from build123d import *

# Parameters (mm, degrees)
SKIZZE1_W                       = 730
SKIZZE1_H                       = 1060
AUFSATZ_LINEAR_AUSTRAGEN1_DEPTH = 21
SKIZZE2_W                       = 17
SKIZZE2_H                       = 1060
SCHNITT_LINEAR_AUSTRAGEN1_DEPTH = 11
SKIZZE3_R                       = 3.5
SCHNITT_LINEAR_AUSTRAGEN2_DEPTH = 40


with BuildPart() as part:
    # Skizze1 → Aufsatz-Linear austragen1 (new body)
    with BuildSketch(Plane.XY):
        Rectangle(SKIZZE1_W, SKIZZE1_H)
    extrude(amount=AUFSATZ_LINEAR_AUSTRAGEN1_DEPTH)

    # Skizze2 → Schnitt-Linear austragen1 (cut)
    with BuildSketch(Plane.XY.offset(21)):
        with Locations((58.5, 0)):
            Rectangle(SKIZZE2_W, SKIZZE2_H)
        with Locations((175.5, 0)):
            Rectangle(SKIZZE2_W, SKIZZE2_H)
        with Locations((292.5, 0)):
            Rectangle(SKIZZE2_W, SKIZZE2_H)
        with Locations((-292.5, 0)):
            Rectangle(SKIZZE2_W, SKIZZE2_H)
        with Locations((-175.5, 0)):
            Rectangle(SKIZZE2_W, SKIZZE2_H)
        with Locations((-58.5, 0)):
            Rectangle(SKIZZE2_W, SKIZZE2_H)
    extrude(amount=-SCHNITT_LINEAR_AUSTRAGEN1_DEPTH, mode=Mode.SUBTRACT)

    # Skizze3 → Schnitt-Linear austragen2 (cut)
    with BuildSketch(Plane.XY.offset(21)):
        with Locations((0, 490)):
            Circle(SKIZZE3_R)
        with Locations((117, 490)):
            Circle(SKIZZE3_R)
        with Locations((234, 490)):
            Circle(SKIZZE3_R)
        with Locations((340, 490)):
            Circle(SKIZZE3_R)
        with Locations((340, 190)):
            Circle(SKIZZE3_R)
        with Locations((234, 190)):
            Circle(SKIZZE3_R)
        with Locations((117, 190)):
            Circle(SKIZZE3_R)
        with Locations((0, 190)):
            Circle(SKIZZE3_R)
        with Locations(Location((-340, 490, 0), (0, 0, 180))):
            Circle(SKIZZE3_R)
        with Locations(Location((-234, 490, 0), (0, 0, 180))):
            Circle(SKIZZE3_R)
        with Locations(Location((-117, 490, 0), (0, 0, 180))):
            Circle(SKIZZE3_R)
    extrude(amount=-SCHNITT_LINEAR_AUSTRAGEN2_DEPTH, mode=Mode.SUBTRACT)


solid = part.part
Can you work these out from the model? Positions are in its coordinate system, mm. Round coordinates to 2 decimals unless told otherwise and drop trailing zeros. Write each loop counter-clockwise with the first axis right and the second up, starting at its lowest first coordinate (ties: lowest second). Pieces come first, ordered by that corner, then holes. Notation, with made-up numbers: M 18,29.25 L 27,29.25 A18 ccw 27,51.25 Z; hole C 27,-14 d2. An arc over 180 degrees is marked long. Use CSV: the item, a comma, the result in double quotes.
(1) I need wall thicknesses on line 1 along Y through (x, z) = (117, 15.5); line 2 along Y through (x, z) = (-234, 6.75); line 3 along Y through (x, z) = (-1.5, 9.5). Which ranges of each line are inside material? Lowest first, please.
Check values:
line 1,"-530 to 186.5, 193.5 to 486.5, 493.5 to 530"
line 2,"-530 to 486.5, 493.5 to 530"
line 3,"-530 to 186.84, 193.16 to 486.84, 493.16 to 530"
(2) Imagine slicing it at B-B (y = -337). Write out the boundary of the cut face in (x, z), plus the area to 3 significant figures.
Check values:
outline,"M -365,0 L 365,0 L 365,21 L 301,21 L 301,10 L 284,10 L 284,21 L 184,21 L 184,10 L 167,10 L 167,21 L 67,21 L 67,10 L 50,10 L 50,21 L -50,21 L -50,10 L -67,10 L -67,21 L -167,21 L -167,10 L -184,10 L -184,21 L -284,21 L -284,10 L -301,10 L -301,21 L -365,21 Z"
area,"14,200 mm^2"
(3) I'm going to push a flat-ended pin straight in: pin 1 (5 mm diameter, centred on x = 62, y = -173.5, fed in from +Z). Where does the tip first touch, or does it pass through?
Check values:
pin 1,"z = 10"
(4) Imagine slicing it at A-A (z = 16.25). Count the separate pieces of the cut face and the enclosed holes in it, plus the area to 3 significant figures.
Check values:
separate pieces,"7"
enclosed holes,"11"
area,"665,000 mm^2"
